from build123d import *

# Parameters (mm, degrees)
F1_DEPTH    = 2.75
F3_DEPTH    = 16.7
F4_C1_SIZE2 = 2.852938746
F4_C1_SIZE  = 3.4
F4_C2_SIZE2 = 2.852938746
F4_C2_SIZE  = 3.4


with BuildPart() as f1:
    # F0 (on Top) → F1 (new body, symmetric)
    with BuildSketch(Plane.XY):
        Polygon((9.15, 81.3), (0, 81.3), (-9.15, 81.3), (-9.15, 37.3), (-51.8, 37.3), (-51.8, 18.8), (-9.15, 18.8), (-9.15, -81.2), (0, -81.2), (9.15, -81.2), (9.15, 18.8), (52.55, 18.8), (52.55, 37.3), (9.15, 37.3), align=None)
    extrude(amount=F1_DEPTH, both=True)

    # F2 (on Right) → F3 (join, symmetric)
    with BuildSketch(Plane.YZ):
        Polygon((-74.0734412255, -10.8967302314), (-74, -2.75), (-73.8589504462, 12.8964254994), (-77.2330946452, 15.7798974367), (-81.3329280584, 15.8168566562), (-81.4996952681, -2.6823916718), (-81.5988541495, -13.6819447316), (-77.4990207363, -13.718903951), align=None)
    extrude(amount=F3_DEPTH, both=True)

    # F4: chamfer of 3.4 x 2.852938746 on 2 edges, made by hand

    # F4_c1
    f4_c1_edges = [f1.edges().sort_by_distance(p)[0] for p in [
        (-16.7, -73.9661958359, 0.999847634),
    ]]
    f4_c1_side = f1.faces().sort_by_distance((-16.6429412251, -73.9661958359, 0.999847634))[0]
    chamfer(f4_c1_edges, length=F4_C1_SIZE, length2=F4_C1_SIZE2, reference=f4_c1_side)

    # F4_c2
    f4_c2_edges = [f1.edges().sort_by_distance(p)[0] for p in [
        (16.7, -73.9661958359, 0.999847634),
    ]]
    f4_c2_side = f1.faces().sort_by_distance((16.6429412251, -73.9661958359, 0.999847634))[0]
    chamfer(f4_c2_edges, length=F4_C2_SIZE, length2=F4_C2_SIZE2, reference=f4_c2_side)


solid = f1.part
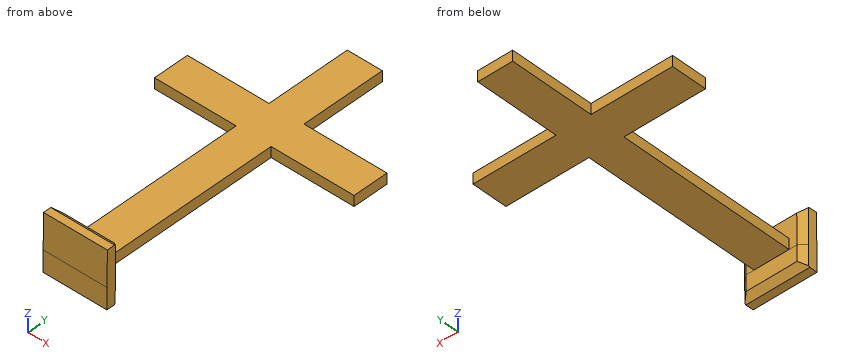
CAD build for the part. Positions are in the model's coordinates, mm. Round coordinates to 2 decimals unless told otherwise and drop trailing zeros. Write each loop counter-clockwise with the first axis right and the second up, starting at its lowest first coordinate (ties: lowest second). Pieces come first, ordered by that corner, then holes.
(1) Drop flat-ended pins along their axis: P1, Ø10, axis at x = -16, y = 4.5, coming from the -Z side; P2, Ø1.5, axis at y = -79, z = 3, coming from the -X side; P3, Ø4.5, axis at y = -4.5, z = -1, coming from the -X side; P4, Ø5, axis at x = 14, y = 39, coming from the -Z side. Give the stop position or say it passes through.
(2) Slice it at C-C, the plane y = 4.5. Write the cut outline in (x, z).
(3) Probe line 1 along Y through (x, z) = (27.5, -2.5); line 2 along Y through (x, z) = (-3.5, -2.25); line 3 along X through (y, z) = (-4, -1.75). List the from-to ranges inside material, lowest first.
(4) Slice it at A-A, the plane x = -1. Write the cut outline in (y, z), and give its area (3 significant figures).
(5) Slice it at D-D, the plane x = -26.5. Write the cut outline in (y, z), and give its area (3 significant figures).
(6) Slice it at B-B, the plane z = -0.5. Write the cut outline in (x, y).
From the geometry:
1. P1: passes through
1. P2: stops at x = -16.7
1. P3: stops at x = -9.15
1. P4: stops at z = -2.75
2. outline: (-9.15, -2.75) - (9.15, -2.75) - (9.15, 2.75) - (-9.15, 2.75) - close
3. line 1: y = 18.8 to 37.3
3. line 2: y = -81.5 to 81.3
3. line 3: x = -9.15 to 9.15
4. outline: (-81.6, -13.68) - (-77.5, -13.72) - (-74.07, -10.9) - (-74, -2.75) - (81.3, -2.75) - (81.3, 2.75) - (-73.95, 2.75) - (-73.86, 12.9) - (-77.23, 15.78) - (-81.33, 15.82) - close
4. area: 1,070 mm2
5. outline: (18.8, -2.75) - (37.3, -2.75) - (37.3, 2.75) - (18.8, 2.75) - close
5. area: 102 mm2
6. outline: (-51.8, 18.8) - (-9.15, 18.8) - (-9.15, -73.98) - (-13.3, -73.98) - (-16.7, -76.83) - (-16.7, -81.48) - (16.7, -81.48) - (16.7, -76.83) - (13.3, -73.98) - (9.15, -73.98) - (9.15, 18.8) - (52.55, 18.8) - (52.55, 37.3) - (9.15, 37.3) - (9.15, 81.3) - (-9.15, 81.3) - (-9.15, 37.3) - (-51.8, 37.3) - close
